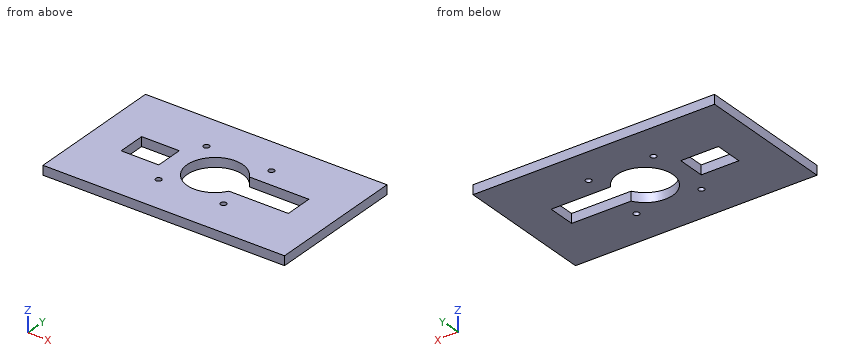
Autodesk Inventor part; units mm, degrees
ref_plane "YZ Plane" through (0, 0, 0) normal (1, 0, 0) x (0, 1, 0)
ref_plane "XZ Plane" through (0, 0, 0) normal (0, 1, 0) x (-1, 0, 0)
ref_plane "XY Plane" through (0, 0, 0) normal (0, 0, 1) x (1, 0, 0)
sketch "Skizze2" plane through (0, 0, 0) normal (0, 0, 1) x (1, 0, 0)
  line L0 (145, 0) -> (260, 0)
  line L1 (260, 0) -> (260, 150)
  line L2 (260, 150) -> (0, 150)
  line L3 (0, 150) -> (0, 0)
  line L4 (0, 0) -> (145, 0)
  circle A0 centre (165.0018, 110.0018) radius 3.1
  circle A1 centre (165.0018, 39.9982) radius 3.1
  circle A2 centre (94.9982, 39.9982) radius 3.1
  circle A3 centre (94.9982, 110.0018) radius 3.1
  arc A4 (155.9808, 90) -> (155.9808, 60) centre (130, 75) ccw
  line L5 (155.9808, 90) -> (220, 90)
  line L6 (220, 90) -> (220, 60)
  line L7 (220, 60) -> (155.9808, 60)
  line L8 (40, 90) -> (80.5, 90)
  line L9 (80.5, 90) -> (80.5, 60)
  line L10 (80.5, 60) -> (40, 60)
  line L11 (40, 60) -> (40, 90)
  dimension "d13" = 6.2
  dimension "d14" = 30
  dimension "d15" = 90
  dimension "d16" = 90
  dimension "d17" = 90
  dimension "d18" = 40
  dimension "d19" = 179.5
  dimension "d20" = 220
  dimension "d21" = 260
  dimension "d22" = 150
  dimension "d23" = 60
  dimension "d24" = 90
  dimension "d25" = 260
  dimension "d26" = 0
  dimension "d27" = 90
  dimension "d28" = 60
  dimension "d29" = 150
  dimension "d30" = 150
  dimension "d31" = 0
  dimension "d32" = 0
  dimension "d33" = 150
  dimension "d34" = 0
  dimension "d35" = 0
  dimension "d36" = 0
  dimension "d37" = 0
  dimension "d38" = 90
  dimension "d39" = 40
  dimension "d40" = 40
  dimension "d41" = 90
  dimension "d42" = 60
  dimension "d43" = 40
  dimension "d44" = 40
  dimension "d45" = 60
  dimension "d46" = 94.9982
  dimension "d47" = 110.0018
  dimension "d48" = 94.9982
  dimension "d49" = 39.9982
  dimension "d50" = 104.0192
  dimension "d51" = 104.0192
  dimension "d52" = 115
  dimension "d53" = 115
  dimension "d54" = 115
  dimension "d55" = 0
  dimension "d56" = 165.0018
  dimension "d57" = 110.0018
  dimension "d58" = 165.0018
  dimension "d59" = 39.9982
  dimension "d60" = 90
  dimension "d61" = 179.5
  dimension "d62" = 179.5
  dimension "d63" = 90
  dimension "d64" = 60
  dimension "d65" = 179.5
  dimension "d66" = 179.5
  dimension "d67" = 30
  dimension "d68" = 90
  dimension "d69" = 220
  dimension "d70" = 220
  dimension "d71" = 90
  dimension "d72" = 60
  dimension "d73" = 220
  dimension "d74" = 220
  dimension "d75" = 60
  dimension "d76" = 150
extrude "Extrusion1" add sketch "Skizze2" along normal blind 10
properties part number "MotorHalterung"
Build history of the part. All positions in model axes, mm. Give positions to 0.01 mm unless a question says otherwise; leave off trailing zeros. Loops run counter-clockwise (first coordinate to the right, second up) from the corner with the lowest first, then second, coordinate; pieces in that order, holes last. Notation, with made-up numbers: (6, -32) - (27, -32) arc R27 cw to (27, -9) - close; hole circle Ø11 at (82.25, 60). An arc over 180 degrees is marked (long way). Use a Markdown table: item, result.
(1) Wall check: line 1 along X through (y, z) = (75, 4.25); line 2 along Y through (x, z) = (46, 3.25); line 3 along X through (y, z) = (69.5, 8.5). Give the ranges that are in metal, low to high.
Taken from the geometry:
| item | result |
|---|---|
| line 1 | 0 to 40, 80.5 to 100, 220 to 260 |
| line 2 | 0 to 60, 90 to 150 |
| line 3 | 0 to 40, 80.5 to 100.51, 220 to 260 |
(2) Drop flat-ended pins along their axis: pin 1 Ø5.5 at (x, y) = (165, 110) entering from +Z; pin 2 Ø3 at (y, z) = (75, 4.5) entering from -X. Give the stop position or say it passes through.
Taken from the geometry:
| item | result |
|---|---|
| pin 1 | through |
| pin 2 | x = 0 |
(3) Band-saw the part on B-B (y = 75). Give the cut face in (x, z).
Taken from the geometry:
| item | result |
|---|---|
| outline | (0, 0) - (40, 0) - (40, 10) - (0, 10) - close; (80.5, 0) - (100, 0) - (100, 10) - (80.5, 10) - close; (220, 0) - (260, 0) - (260, 10) - (220, 10) - close |
(4) Band-saw the part on A-A (x = 130). Give the cut face in (y, z).
Taken from the geometry:
| item | result |
|---|---|
| outline | (0, 0) - (45, 0) - (45, 10) - (0, 10) - close; (105, 0) - (150, 0) - (150, 10) - (105, 10) - close |
(5) Band-saw the part on C-C (z = 1.5). Give the cut face in (x, y).
Taken from the geometry:
| item | result |
|---|---|
| outline | (0, 0) - (260, 0) - (260, 150) - (0, 150) - close; hole (40, 60) - (80.5, 60) - (80.5, 90) - (40, 90) - close; hole circle Ø6.2 at (95, 40); hole circle Ø6.2 at (95, 110); hole (155.98, 60) - (220, 60) - (220, 90) - (155.98, 90) arc R30 ccw (long way) to start; hole circle Ø6.2 at (165, 40); hole circle Ø6.2 at (165, 110) |
